```python
from build123d import *

# Parameters (mm, degrees)
F1_DEPTH = 200
F2_W     = 335.056305
F2_H     = 699.782848
F3_DEPTH = 330.21611


with BuildPart() as f1:
    # F0 (on Right) → F1 (new body, symmetric)
    with BuildSketch(Plane.YZ):
        with BuildLine():
            ThreePointArc((851.475526, 116.391551), (739.643276, 223.843098), (627.811026, 116.391551))
            Line((627.811026, 116.391551), (851.475526, 116.391551))
        make_face()
        with BuildLine():
            ThreePointArc((10.594565, 112.123632), (122.41489, 4.6e-05), (234.437481, 111.921549))
            ThreePointArc((234.437481, 111.921549), (234.415154, 114.156996), (234.348182, 116.391551))
            Line((234.348182, 116.391551), (10.594565, 112.123632))
        make_face()
        with BuildLine():
            Line((10.594565, 112.123632), (234.348182, 116.391551))
            ThreePointArc((234.348182, 116.391551), (120.381507, 223.822743), (10.594565, 112.123632))
        make_face()
        with BuildLine():
            Line((851.475526, 116.391551), (627.811026, 116.391551))
            ThreePointArc((627.811026, 116.391551), (737.407829, 0.022327), (851.564825, 111.921549))
            ThreePointArc((851.564825, 111.921549), (851.542498, 114.156996), (851.475526, 116.391551))
        make_face()
        with BuildLine():
            ThreePointArc((10.594565, 112.123632), (120.381507, 223.822743), (234.348182, 116.391551))
            Line((234.348182, 116.391551), (627.811026, 116.391551))
            ThreePointArc((627.811026, 116.391551), (739.643276, 223.843098), (851.475526, 116.391551))
            Line((851.475526, 116.391551), (1208.921194, 204.149604))
            Line((1208.921194, 204.149604), (1208.921194, 562.703967))
            Line((1208.921194, 562.703967), (620.193636, 402.439284))
            Line((620.193636, 402.439284), (578.239322, 391.018391))
            Line((578.239322, 391.018391), (133.258164, 343.13333))
            Line((133.258164, 343.13333), (0, 194.806337))
            Line((0, 194.806337), (0, 111.921549))
            Line((0, 111.921549), (10.594565, 112.123632))
        make_face()
        Polygon((988.866329, 900), (578.239322, 391.018391), (620.193636, 402.439284), (988.866329, 859.417558), (1250, 859.417558), (1250, 900), align=None)
    extrude(amount=F1_DEPTH, both=True)

    # F2 (on face) → F3 (cut)
    with BuildSketch(Plane.XY.offset(900)):
        with Locations((-0.824928, 858.516693)):
            Rectangle(F2_W, F2_H)
    extrude(amount=-F3_DEPTH, mode=Mode.SUBTRACT)


solid = f1.part
```
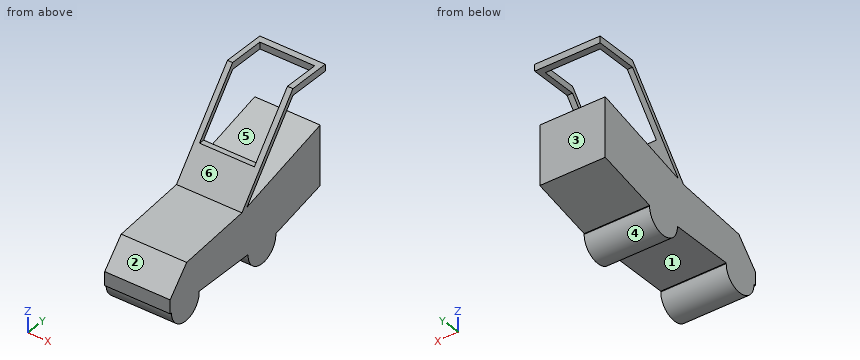
The model under review builds one solid part; all positions refer to its coordinate system, in mm. Face numbers are marked on the shaded views. A direction names the side the tool comes from. Give positions to 0.01 mm unless a question says otherwise; leave off trailing zeros. Write each loop counter-clockwise with the first axis right and the second up, starting at its lowest first coordinate (ties: lowest second). Pieces come first, ordered by that corner, then holes.
(1) Consider section B-B, the plane z = 68.5. Give the boundary of the cut face in (x, y), and give its area (3 significant figures).
(2) Consider section D-D, the plane z = 522. Give the boundary of the cut face in (x, y), and give its area (3 significant figures).
(3) Tool access review of the marked faces 1 and 2: name each direction out of +Z, -Z, +X, -X, +Y, -Y from which nothing blocks a thin tool from reaching the whole face with its end or side.
(4) Consider section A-A, the plane x = -88.5. Give the boundary of the cut face in (y, z).
(5) For P1, Ø3, axis at x = 110, y = 761, coming from the +Z side; P2, Ø1, axis at x = -138.5, z = 223.5, coming from the -Y side; P3, Ø6, axis at x = -87.5, z = 469, coming from the -Y side, all flat-tipped, find the tip position at first contact; note any pin that passes through.
(6) To check wall thickness, follow L1, parallel to Y at x = 20, z = 108.5; L2, parallel to Z at x = 11, y = 644.5; L3, parallel to Z at x = -18.5, y = 665.5. State the ranges of each line that lie inside material, in increasing order.
(7) Consider section C-C, the plane y = 1064.5. Give the boundary of the cut face in (x, z).
(8) The part is to be moulded in two halves that separate along Y. For the marked faces 3, 4, 5 and 6, say which applies: released by +Y, released by -Y, zero draft, split by the parting line, or undercut.
Returned:
1. outline: (-200, 19.36) - (200, 19.36) - (200, 225.67) - (-200, 225.67) - close; (-200, 636.49) - (200, 636.49) - (200, 842.8) - (-200, 842.8) - close
1. area: 165,000 mm2
2. outline: (-200, 683.91) - (200, 683.91) - (200, 716.65) - (-200, 716.65) - close; (-200, 1059.4) - (200, 1059.4) - (200, 1208.92) - (-200, 1208.92) - close
2. area: 72,900 mm2
3. face 1: -Z, +X, -X
3. face 2: +Z, +X, -X, -Y
4. outline: (0, 111.92) - (10.59, 112.12) arc R111.92 ccw to (234.44, 111.92) arc R111.92 ccw to (234.35, 116.39) - (627.81, 116.39) arc R111.92 ccw (long way) to (851.56, 111.92) arc R111.92 ccw to (851.48, 116.39) - (1208.92, 204.15) - (1208.92, 562.7) - (620.19, 402.44) - (755.2, 569.78) - (722.46, 569.78) - (578.24, 391.02) - (133.26, 343.13) - (0, 194.81) - close; (1208.41, 859.42) - (1250, 859.42) - (1250, 900) - (1208.41, 900) - close
5. P1: stops at z = 441.18
5. P2: stops at y = 25.33
5. P3: stops at y = 638.73
6. L1: y = 10.65 to 234.39, 627.77 to 851.51
6. L2: z = 52.98 to 409.06, 432.57 to 473.15
6. L3: z = 28.08 to 414.77, 458.6 to 499.18
7. outline: (-200, 168.69) - (200, 168.69) - (200, 523.39) - (-200, 523.39) - close; (-200, 859.42) - (-168.35, 859.42) - (-168.35, 900) - (-200, 900) - close; (166.7, 859.42) - (200, 859.42) - (200, 900) - (166.7, 900) - close
8. face 3: released by +Y
8. face 4: undercut
8. face 5: undercut
8. face 6: released by -Y
